Geometry check sheet. Reference: the model listing, model coordinates, mm. A direction names the side the tool comes from. Give positions to 0.01 mm unless a question says otherwise; leave off trailing zeros. Write each loop counter-clockwise with the first axis right and the second up, starting at its lowest first coordinate (ties: lowest second). Pieces come first, ordered by that corner, then holes. Notation, with made-up numbers: (33, 82.25) - (77, 82.25) arc R27 cw to (77, 116.25) - close; hole circle Ø1 at (35.25, 33). An arc over 180 degrees is marked (long way). Use a Markdown table: item, result.
```python
from build123d import *

# Parameters (mm, degrees)
F1_DEPTH = 2438.4
F3_D     = 13.4874


with BuildPart() as f1:
    # F0 (on Front) → F1 (new body)
    with BuildSketch(Plane.XZ):
        Polygon((-57.316309, 46.347476), (-63.666309, 46.347476), (-63.666309, -29.852524), (12.533691, -29.852524), (12.533691, -23.502524), (-57.316309, -23.502524), align=None)
    extrude(amount=F1_DEPTH)

    # F3 (through all)
    with Locations(Plane(origin=(-63.666309, 0, 0), x_dir=(0, -1, 0), z_dir=(-1, 0, 0))):
        with Locations((2336.8, 14.597476), (2133.6, 14.597476), (1930.4, 14.597476), (1727.2, 14.597476), (1524, 14.597476), (1320.8, 14.597476), (1117.6, 14.597476), (914.4, 14.597476), (711.2, 14.597476), (508, 14.597476), (304.8, 14.597476), (101.6, 14.597476)):
            Hole(F3_D / 2)


solid = f1.part
```
1) Set-up check for faces 1 (the flat face through (-57.316, -1202, 11)), 2 (the flat face through (-63.666, -1202, 9)): record each of +Z, -Z, +X, -X, +Y, -Y from which the full face is reachable in a straight line by a thin tool's end or side.
Working result:
| item | result |
|---|---|
| face 1 | +Z, +X, +Y, -Y |
| face 2 | +Z, -Z, -X, +Y, -Y |
2) Material ranges on L1, parallel to Z at x = -59.5, y = -1320.8; L2, parallel to Z at x = -39.5, y = -1429.5; L3, parallel to X at y = -344.5, z = 34.5, recorded low to high. Write a range as from..to.
Working result:
| item | result |
|---|---|
| L1 | z = -29.85..7.85, 21.34..46.35 |
| L2 | z = -29.85..-23.5 |
| L3 | x = -63.67..-57.32 |
3) Section check A-A on y = -453. Record the boundary of the cut face in (x, z).
Working result:
| item | result |
|---|---|
| outline | (-63.67, -29.85) - (12.53, -29.85) - (12.53, -23.5) - (-57.32, -23.5) - (-57.32, 46.35) - (-63.67, 46.35) - close |
4) Section check B-B on x = -14. Record the boundary of the cut face in (y, z), then the cut area to 3 significant figures.
Working result:
| item | result |
|---|---|
| outline | (-2438.4, -29.85) - (0, -29.85) - (0, -23.5) - (-2438.4, -23.5) - close |
| area | 15,500 mm² |
5) Depth check by flat-ended pin: P1, Ø10, axis at x = -48.5, y = -390, coming from the +Z side; P2, Ø15.5, axis at y = -1320.8, z = 14.6, coming from the +X side. Enter the tip coordinate at first touch or a pass-through.
Working result:
| item | result |
|---|---|
| P1 | stops at z = -23.5 |
| P2 | stops at x = -57.32 |
